```python
from build123d import *

# Parameters (mm, degrees)
F0_W      = 30.2820764482
F0_H      = 101.4822497964
F3_DEPTH  = 25.4
F2_R      = 15.0499216081
F4_DEPTH  = 25.4
F1_R      = 15.5943038306
F5_DEPTH  = 25.4
F6_R      = 10.2440117392
F7_DEPTH  = 49.022
F8_R      = 10.3251238381
F9_DEPTH  = 31.75
F10_W     = 15.6584940851
F10_H     = 42.4823574722
F11_DEPTH = 20.066
F12_R     = 13.1812227962
F13_DEPTH = 25.4
F14_DEPTH = 25.4
F16_DEPTH = 8.128
F18_DEPTH = 7.874
F19_R     = 4.4761775303
F20_DEPTH = 55.118


with BuildPart() as f3:
    # F0 (on Top) → F3 (new body)
    with BuildSketch(Plane.XY):
        Rectangle(F0_W, F0_H)
    extrude(amount=F3_DEPTH)

    # F2 (on Top) → F4 (join)
    with BuildSketch(Plane.XY):
        with Locations((0, -51.2032657862)):
            Circle(F2_R)
    extrude(amount=F4_DEPTH)

    # F1 (on Top) → F5 (join)
    with BuildSketch(Plane.XY):
        with Locations((0, 50.4214018583)):
            Circle(F1_R)
    extrude(amount=F5_DEPTH)

    # F6 (on Top) → F7 (cut)
    with BuildSketch(Plane.XY):
        with Locations((0, 51.5931844711)):
            Circle(F6_R)
    extrude(amount=F7_DEPTH, mode=Mode.SUBTRACT)

    # F8 (on Top) → F9 (cut)
    with BuildSketch(Plane.XY):
        with Locations((0, -48.5663115978)):
            Circle(F8_R)
    extrude(amount=F9_DEPTH, mode=Mode.SUBTRACT)

    # F10 (on Top) → F11 (join)
    with BuildSketch(Plane.XY):
        Rectangle(F10_W, F10_H)
    extrude(amount=-F11_DEPTH)

    # F12 (on Right) → F13 (cut)
    with BuildSketch(Plane.YZ):
        with Locations((0, -18.9247615635)):
            Circle(F12_R)
    extrude(amount=-F13_DEPTH, mode=Mode.SUBTRACT)

    # F14 (cut): a face of the model
    f14_faces = [f3.faces().sort_by_distance(p)[0] for p in [
        (0, 0, -13.9418780745),
    ]]
    extrude(f14_faces, amount=-F14_DEPTH, mode=Mode.SUBTRACT)

    # F15 (on face) → F16 (join)
    with BuildSketch(Plane(origin=(0, 21.2411787361, 0), x_dir=(-1, 0, 0), z_dir=(0, 1, 0))):
        with BuildLine():
            ThreePointArc((-7.4920039842, -20.066), (0, -27.5580039842), (7.4920039842, -20.066))
            Line((7.4920039842, -20.066), (-7.4920039842, -20.066))
        make_face()
    extrude(amount=-F16_DEPTH)

    # F17 (on face) → F18 (join)
    with BuildSketch(Plane.XZ.offset(21.2411787361)):
        with BuildLine():
            ThreePointArc((-7.8292470425, -18.9932599539), (-0.5376156021, -27.9500884016), (7.9023971338, -20.066))
            ThreePointArc((7.9023971338, -20.066), (7.8840884016, -19.5283843979), (7.8292470425, -18.9932599539))
            Line((7.8292470425, -18.9932599539), (7.8292470425, -20.066))
            Line((7.8292470425, -20.066), (-7.8292470425, -20.066))
            Line((-7.8292470425, -20.066), (-7.8292470425, -18.9932599539))
        make_face()
    extrude(amount=-F18_DEPTH)

    # F19 (on face) → F20 (cut)
    with BuildSketch(Plane.XZ.offset(21.2411787361)):
        with Locations((0, -20.066)):
            Circle(F19_R)
    extrude(amount=-F20_DEPTH, mode=Mode.SUBTRACT)


solid = f3.part
```
Source: CAD feature listing. Evaluate the final solid. Frame: model axes, mm. A direction names the side the tool comes from. Coordinates: 2 decimals unless noted, no trailing zeros. Loops run counter-clockwise (first coordinate to the right, second up) from the corner with the lowest first, then second, coordinate; pieces in that order, holes last. Notation, with made-up numbers: M 29.5,34.5 L 75.5,34.5 A18 cw 75.5,69.5 Z; hole C 76,-29.75 d3. An arc over 180 degrees is marked long. Put each result on its own line as item: value. Start each with the question number.
1) Reachability of faces 1 (the face through (0, 13.113, -25)), 2 (the face through (0, -21.241, -11)), 3 (the face through (15.141, -3, 13)) from +Z, -Z, +X, -X, +Y, -Y: full face, straight path, thin tool, end or side. Return the list, or none.
2) Contact query for flat-ended pins moving along their axis: pin 1 Ø4.5 at (x, z) = (2, -18.5) entering from -Y; pin 2 Ø8 at (x, z) = (-8, 19.5) entering from +Y; pin 3 Ø6 at (y, z) = (35, 0.5) entering from -X; pin 4 Ø18.5 at (x, y) = (0, 51.59) entering from -Z. Output: stop coordinate, or through.
3) Cut plane C-C on z = 17. Return the cut outline in (x, y), then the cut area to 3 significant figures.
4) Pull-direction query (Y, two-part tool) for faces 4 (the face through (0, -13.367, -25)), 5 (the face through (-11, 1, 0)), 6 (the face through (-2.221, 41.593, 12.522)), 7 (the face through (0.4, 66.01, 12.52)); classes: pulls with the +Y half, pulls with the -Y half, needs draft (parallel to the pull), parting line crosses it, or undercut.
5) Cut plane B-B on y = 0. Return the cut outline in (x, z), then the cut area to 3 significant figures.
6) Cut plane A-A on x = 0. Return the cut outline in (y, z), then the cut area to 3 significant figures.
7) Cut plane D-D on y = -30. Return the cut outline in (x, z), then the cut area to 3 significant figures.
8) Ray query, L1, parallel to Y at x = 0, z = 6.5; L2, parallel to Y at x = -6.5, z = 2; L3, parallel to Y at x = 6, z = -4. Return the intervals inside material, ascending. Write a range as from..to.
The answers:
1. face 1: -Z, +X, -X
1. face 2: -Z, +X, -X, -Y
1. face 3: +Z, -Z, +X, -Y
2. pin 1: stops at y = -21.24
2. pin 2: stops at y = 65.49
2. pin 3: stops at x = -15.14
2. pin 4: passes through
3. outline: M -15.14,-50.74 L -15.04,-50.74 A15.05 ccw long 15.04,-50.74 L 15.14,-50.74 L 15.14,46.69 A15.59 ccw long -15.14,46.69 Z; hole C 0,-48.57 d20.65; hole C 0,51.59 d20.49
3. area: 3,150 mm²
4. face 4: undercut
4. face 5: needs draft
4. face 6: undercut
4. face 7: parting line crosses it
5. outline: M -15.14,0 L -7.83,0 L -7.83,-5.74 L 7.83,-5.74 L 7.83,0 L 15.14,0 L 15.14,25.4 L -15.14,25.4 Z
5. area: 859 mm²
6. outline: M -66.25,0 L -58.89,0 L -58.89,25.4 L -66.25,25.4 Z; M -38.24,0 L -21.24,0 L -21.24,-15.59 L -12.75,-15.59 A13.18 cw 12.75,-15.59 L 21.24,-15.59 L 21.24,0 L 41.35,0 L 41.35,25.4 L -38.24,25.4 Z; M -21.24,-27.97 L -13.37,-27.97 L -13.37,-24.54 L -21.24,-24.54 Z; M 13.11,-27.56 L 21.24,-27.56 L 21.24,-24.54 L 13.11,-24.54 Z; M 61.84,0 L 66.02,0 L 66.02,25.4 L 61.84,25.4 Z
6. area: 2,840 mm²
7. outline: M -15.14,0 L 15.14,0 L 15.14,25.4 L -15.14,25.4 Z
7. area: 769 mm²
8. L1: y = -66.25..-58.89, -38.24..41.35, 61.84..66.02
8. L2: y = -64.78..-56.59, -40.54..43.68, 59.51..64.6
8. L3: y = -21.24..21.24
